from build123d import *

# Parameters (mm, degrees)
F2_DEPTH = 279.4


with BuildPart() as f2:
    # F1 (on Front) → F2 (new body)
    with BuildSketch(Plane.XZ):
        with BuildLine():
            Line((-0.127, 13.335), (88.9, 13.335))
            Line((88.9, 13.335), (177.927, 13.335))
            Line((177.927, 13.335), (177.927, 13.775847))
            Line((177.927, 13.775847), (177.927, 15.642254))
            Line((177.927, 15.642254), (177.662522, 43.743075))
            ThreePointArc((177.662522, 43.743075), (177.214221, 44.804123), (176.149, 45.242418))
            ThreePointArc((176.149, 45.242418), (175.083779, 44.804123), (174.635478, 43.743075))
            Line((174.635478, 43.743075), (174.371, 15.642254))
            ThreePointArc((174.371, 15.642254), (172.9105, 14.195435), (171.45, 15.642254))
            Line((171.45, 15.642254), (171.12614, 50.052427))
            ThreePointArc((171.12614, 50.052427), (170.695427, 51.071846), (169.672, 51.492945))
            ThreePointArc((169.672, 51.492945), (168.648573, 51.071846), (168.21786, 50.052427))
            Line((168.21786, 50.052427), (167.894, 15.642254))
            ThreePointArc((167.894, 15.642254), (166.4335, 14.195435), (164.973, 15.642254))
            Line((164.973, 15.642254), (164.586194, 56.74034))
            ThreePointArc((164.586194, 56.74034), (164.174126, 57.715632), (163.195, 58.118503))
            ThreePointArc((163.195, 58.118503), (162.215874, 57.715632), (161.803806, 56.74034))
            Line((161.803806, 56.74034), (161.417, 15.642254))
            ThreePointArc((161.417, 15.642254), (159.9565, 14.195435), (158.496, 15.642254))
            Line((158.496, 15.642254), (158.052188, 62.797323))
            ThreePointArc((158.052188, 62.797323), (157.657005, 63.73265), (156.718, 64.119013))
            ThreePointArc((156.718, 64.119013), (155.778995, 63.73265), (155.383812, 62.797323))
            Line((155.383812, 62.797323), (154.94, 15.642254))
            ThreePointArc((154.94, 15.642254), (153.4795, 14.195435), (152.019, 15.642254))
            Line((152.019, 15.642254), (151.511, 69.617254))
            ThreePointArc((151.511, 69.617254), (150.241, 70.887254), (148.971, 69.617254))
            Line((148.971, 69.617254), (148.463, 15.642254))
            ThreePointArc((148.463, 15.642254), (147.0025, 14.195435), (145.542, 15.642254))
            Line((145.542, 15.642254), (145.034, 69.617254))
            ThreePointArc((145.034, 69.617254), (143.764, 70.887254), (142.494, 69.617254))
            Line((142.494, 69.617254), (141.986, 15.642254))
            ThreePointArc((141.986, 15.642254), (140.5255, 14.195435), (139.065, 15.642254))
            Line((139.065, 15.642254), (138.557, 69.617254))
            ThreePointArc((138.557, 69.617254), (137.287, 70.887254), (136.017, 69.617254))
            Line((136.017, 69.617254), (135.509, 15.642254))
            ThreePointArc((135.509, 15.642254), (134.0485, 14.195435), (132.588, 15.642254))
            Line((132.588, 15.642254), (132.08, 69.617254))
            ThreePointArc((132.08, 69.617254), (130.81, 70.887254), (129.54, 69.617254))
            Line((129.54, 69.617254), (129.032, 15.642254))
            ThreePointArc((129.032, 15.642254), (127.5715, 14.195435), (126.111, 15.642254))
            Line((126.111, 15.642254), (125.603, 69.617254))
            ThreePointArc((125.603, 69.617254), (124.333, 70.887254), (123.063, 69.617254))
            Line((123.063, 69.617254), (122.555, 15.642254))
            ThreePointArc((122.555, 15.642254), (121.0945, 14.195435), (119.634, 15.642254))
            Line((119.634, 15.642254), (119.126, 69.617254))
            ThreePointArc((119.126, 69.617254), (117.856, 70.887254), (116.586, 69.617254))
            Line((116.586, 69.617254), (116.078, 15.642254))
            ThreePointArc((116.078, 15.642254), (114.6175, 14.195435), (113.157, 15.642254))
            Line((113.157, 15.642254), (112.649, 69.617254))
            ThreePointArc((112.649, 69.617254), (111.379, 70.887254), (110.109, 69.617254))
            Line((110.109, 69.617254), (109.601, 15.642254))
            ThreePointArc((109.601, 15.642254), (108.1405, 14.195435), (106.68, 15.642254))
            Line((106.68, 15.642254), (106.172, 69.617254))
            ThreePointArc((106.172, 69.617254), (104.902, 70.887254), (103.632, 69.617254))
            Line((103.632, 69.617254), (103.124, 15.642254))
            ThreePointArc((103.124, 15.642254), (101.6635, 14.195435), (100.203, 15.642254))
            Line((100.203, 15.642254), (99.695, 69.617254))
            ThreePointArc((99.695, 69.617254), (98.425, 70.887254), (97.155, 69.617254))
            Line((97.155, 69.617254), (96.647, 15.642254))
            ThreePointArc((96.647, 15.642254), (95.1865, 14.195435), (93.726, 15.642254))
            Line((93.726, 15.642254), (91.948, 15.642254))
            Line((91.948, 15.642254), (90.17, 15.642254))
            ThreePointArc((90.17, 15.642254), (88.9, 14.384151), (87.63, 15.642254))
            Line((87.63, 15.642254), (85.852, 15.642254))
            Line((85.852, 15.642254), (84.074, 15.642254))
            ThreePointArc((84.074, 15.642254), (82.6135, 14.195435), (81.153, 15.642254))
            Line((81.153, 15.642254), (80.645, 69.617254))
            ThreePointArc((80.645, 69.617254), (79.375, 70.887254), (78.105, 69.617254))
            Line((78.105, 69.617254), (77.597, 15.642254))
            ThreePointArc((77.597, 15.642254), (76.1365, 14.195435), (74.676, 15.642254))
            Line((74.676, 15.642254), (74.168, 69.617254))
            ThreePointArc((74.168, 69.617254), (72.898, 70.887254), (71.628, 69.617254))
            Line((71.628, 69.617254), (71.12, 15.642254))
            ThreePointArc((71.12, 15.642254), (69.6595, 14.195435), (68.199, 15.642254))
            Line((68.199, 15.642254), (67.691, 69.617254))
            ThreePointArc((67.691, 69.617254), (66.421, 70.887254), (65.151, 69.617254))
            Line((65.151, 69.617254), (64.643, 15.642254))
            ThreePointArc((64.643, 15.642254), (63.1825, 14.195435), (61.722, 15.642254))
            Line((61.722, 15.642254), (61.214, 69.617254))
            ThreePointArc((61.214, 69.617254), (59.944, 70.887254), (58.674, 69.617254))
            Line((58.674, 69.617254), (58.166, 15.642254))
            ThreePointArc((58.166, 15.642254), (56.7055, 14.195435), (55.245, 15.642254))
            Line((55.245, 15.642254), (54.737, 69.617254))
            ThreePointArc((54.737, 69.617254), (53.467, 70.887254), (52.197, 69.617254))
            Line((52.197, 69.617254), (51.689, 15.642254))
            ThreePointArc((51.689, 15.642254), (50.2285, 14.195435), (48.768, 15.642254))
            Line((48.768, 15.642254), (48.26, 69.617254))
            ThreePointArc((48.26, 69.617254), (46.99, 70.887254), (45.72, 69.617254))
            Line((45.72, 69.617254), (45.212, 15.642254))
            ThreePointArc((45.212, 15.642254), (43.7515, 14.195435), (42.291, 15.642254))
            Line((42.291, 15.642254), (41.783, 69.617254))
            ThreePointArc((41.783, 69.617254), (40.513, 70.887254), (39.243, 69.617254))
            Line((39.243, 69.617254), (38.735, 15.642254))
            ThreePointArc((38.735, 15.642254), (37.2745, 14.195435), (35.814, 15.642254))
            Line((35.814, 15.642254), (35.306, 69.617254))
            ThreePointArc((35.306, 69.617254), (34.036, 70.887254), (32.766, 69.617254))
            Line((32.766, 69.617254), (32.258, 15.642254))
            ThreePointArc((32.258, 15.642254), (30.7975, 14.195435), (29.337, 15.642254))
            Line((29.337, 15.642254), (28.829, 69.617254))
            ThreePointArc((28.829, 69.617254), (27.559, 70.887254), (26.289, 69.617254))
            Line((26.289, 69.617254), (25.781, 15.642254))
            ThreePointArc((25.781, 15.642254), (24.3205, 14.195435), (22.86, 15.642254))
            Line((22.86, 15.642254), (22.416188, 62.797323))
            ThreePointArc((22.416188, 62.797323), (22.021005, 63.73265), (21.082, 64.119013))
            ThreePointArc((21.082, 64.119013), (20.142995, 63.73265), (19.747812, 62.797323))
            Line((19.747812, 62.797323), (19.304, 15.642254))
            ThreePointArc((19.304, 15.642254), (17.8435, 14.195435), (16.383, 15.642254))
            Line((16.383, 15.642254), (15.996194, 56.74034))
            ThreePointArc((15.996194, 56.74034), (15.584126, 57.715632), (14.605, 58.118503))
            ThreePointArc((14.605, 58.118503), (13.625874, 57.715632), (13.213806, 56.74034))
            Line((13.213806, 56.74034), (12.827, 15.642254))
            ThreePointArc((12.827, 15.642254), (11.3665, 14.195435), (9.906, 15.642254))
            Line((9.906, 15.642254), (9.58214, 50.052427))
            ThreePointArc((9.58214, 50.052427), (9.151427, 51.071846), (8.128, 51.492945))
            ThreePointArc((8.128, 51.492945), (7.104573, 51.071846), (6.67386, 50.052427))
            Line((6.67386, 50.052427), (6.35, 15.642254))
            ThreePointArc((6.35, 15.642254), (4.8895, 14.195435), (3.429, 15.642254))
            Line((3.429, 15.642254), (3.164522, 43.743075))
            ThreePointArc((3.164522, 43.743075), (2.716221, 44.804123), (1.651, 45.242418))
            ThreePointArc((1.651, 45.242418), (0.585779, 44.804123), (0.137478, 43.743075))
            Line((0.137478, 43.743075), (-0.127, 15.642254))
            Line((-0.127, 15.642254), (-0.127, 13.775847))
            Line((-0.127, 13.775847), (-0.127, 13.335))
        make_face()
        Polygon((177.927, 13.335), (88.9, 13.335), (88.9, 0), (177.8, 0), (177.927, 0), align=None)
        Polygon((88.9, 0), (88.9, 13.335), (-0.127, 13.335), (-0.127, 0), (0, 0), align=None)
        with BuildLine():
            Line((91.948, 15.642254), (93.726, 15.642254))
            Line((93.726, 15.642254), (93.218, 69.617254))
            ThreePointArc((93.218, 69.617254), (91.948, 70.887254), (90.678, 69.617254))
            Line((90.678, 69.617254), (90.17, 15.642254))
            Line((90.17, 15.642254), (91.948, 15.642254))
        make_face()
        with BuildLine():
            Line((84.582, 69.617254), (84.074, 15.642254))
            Line((84.074, 15.642254), (85.852, 15.642254))
            Line((85.852, 15.642254), (87.63, 15.642254))
            Line((87.63, 15.642254), (87.122, 69.617254))
            ThreePointArc((87.122, 69.617254), (85.852, 70.887254), (84.582, 69.617254))
        make_face()
    extrude(amount=F2_DEPTH)


solid = f2.part
Build history of the part. All positions in model axes, mm. Round coordinates to 2 decimals unless told otherwise and drop trailing zeros. Use one line per item in the form item = value.
Q1. Drill centre lines: L1, parallel to Z at x = 111, y = -67.5; L2, parallel to Z at x = 95, y = -201.5. Where is each one in solid material? Low to high.
Conclusion:
L1 = 0 to 70.83
L2 = 0 to 14.21
Q2. Band-saw the part on A-A, the plane z = 21. State how many separate pieces and enclosed holes the cut face has, then the cut area to 3 significant figures.
Conclusion:
separate_pieces = 28
enclosed_holes = 0
area = 27,000 mm²
Q3. Drop flat-ended pins along their axis: P1, Ø6, axis at x = 153.5, y = -148.5, coming from the +Z side; P2, Ø1, axis at x = 18, y = -223.5, coming from the +Z side; P3, Ø3, axis at y = -173, z = 36.5, coming from the -X side. Give the stop position or say it passes through.
Conclusion:
P1 = 70.86
P2 = 14.35
P3 = 0.06
